Input: part model. Units: mm. Frame: model coordinates. A direction names the side the tool comes from. Coordinates: 2 decimals unless noted, no trailing zeros. Write each loop counter-clockwise with the first axis right and the second up, starting at its lowest first coordinate (ties: lowest second). Pieces come first, ordered by that corner, then holes. Notation, with made-up numbers: (13.25, 55) - (56.25, 55) arc R17 ccw to (56.25, 69) - close; hole circle Ø10 at (42, -19.75). An arc over 180 degrees is marked (long way). Put each result on its own line as item: value. Start each with the question number.
1. Access query for faces 4 (the flat face through (3, -63.586, -20)), 5 (the flat face through (2.96, -75.19, -37.71)), 6 (the flat face through (3, 14, -11.184)). Directions: +Z, -Z, +X, -X, +Y, -Y. A direction counts if a zero-diameter tool reaches every point of the face in a straight line with its end or side. Return the directions, or none.
2. Cut plane A-A, the plane x = 1.7. Count the separate pieces of the cut face and the enclosed holes in it, and give its area (3 significant figures).
3. Pin query (flat end, axial travel): pin 1 (1.8 mm diameter, centred on x = 1.5, z = -19.5, fed in from +Y); pin 2 (3 mm diameter, centred on x = 3.5, y = -78, fed in from -Z); pin 3 (3 mm diameter, centred on x = 3.5, y = 16.5, fed in from +Z). Return the tip coordinate at first contact, or that it passes through.
4. Cut plane D-D, the plane y = -15.5. Return loops of the section in (x, z).
5. Pull-direction query (Y, two-part tool) for faces 1 (the flat face through (3, -84.98, -9)), 2 (the flat face through (3, -75.586, 4)), 3 (the flat face through (3, 13, -29.184)); classes: released by +Y, released by -Y, zero draft, split by the parting line, or undercut.
6. Cut plane B-B, the plane z = -38. Return loops of the section in (x, y), and give its area (3 significant figures).
7. Line query: line 1 (Y direction, x = 3.5, z = 8.5); line 2 (Z direction, x = 2.75, y = 13); line 3 (Y direction, x = 1.3, z = 14). Output: solid intervals per line, ascending.
8. Cut plane C-C, the plane z = -12.5. Return loops of the section in (x, y), and give its area (3 significant figures).
from build123d import *

# Parameters (mm, degrees)
SKETCH1_W           = 12
SKETCH1_H           = 6
BOSS_EXTRUDE1_DEPTH = 6


with BuildPart() as part:
    # Sketch1 → Boss-Extrude1 (new body)
    with BuildSketch(Plane(origin=(0, 0, 0), x_dir=(0, 0, -1), z_dir=(1, 0, 0))):
        with BuildLine():
            Line((-19.809776263, 10.405108849), (-19.809776263, -84.98038082))
            Line((-19.809776263, -84.98038082), (39.507973257, -84.98038082))
            Line((39.507973257, -84.98038082), (35.862319142, -65.117665917))
            ThreePointArc((35.862319142, -65.117665917), (36.331936953, -30.24496444), (50.023720259, 1.830897499))
            Line((50.023720259, 1.830897499), (52.190223737, 5.008360642))
            Line((52.190223737, 5.008360642), (52.190223737, 10.405108849))
            Line((52.190223737, 10.405108849), (41.184188047, 10.405108849))
            Line((41.184188047, 10.405108849), (41.184188047, 16.405108849))
            Line((41.184188047, 16.405108849), (29.184188047, 16.405108849))
            Line((29.184188047, 16.405108849), (29.184188047, 10.405108849))
            Line((29.184188047, 10.405108849), (11.184188047, 10.405108849))
            Line((11.184188047, 10.405108849), (11.184188047, 18.63698455))
            Line((11.184188047, 18.63698455), (-0.815811953, 18.63698455))
            Line((-0.815811953, 18.63698455), (-0.815811953, 10.405108849))
            Line((-0.815811953, 10.405108849), (-19.809776263, 10.405108849))
        make_face()
        with Locations((-3.863115861, -78.586137139)):
            Rectangle(SKETCH1_W, SKETCH1_H, mode=Mode.SUBTRACT)
        with Locations((20.136884139, -78.586137139)):
            Rectangle(SKETCH1_W, SKETCH1_H, mode=Mode.SUBTRACT)
        with Locations((-3.863115861, -66.586137139)):
            Rectangle(SKETCH1_W, SKETCH1_H, mode=Mode.SUBTRACT)
        with Locations((20.136884139, -66.586137139)):
            Rectangle(SKETCH1_W, SKETCH1_H, mode=Mode.SUBTRACT)
    extrude(amount=BOSS_EXTRUDE1_DEPTH)


solid = part.part
Report:
1. face 4: +X, -X
1. face 5: -Z, +X, -X
1. face 6: +X, -X, +Y
2. separate pieces: 1
2. enclosed holes: 4
2. area: 5,530 mm^2
3. pin 1: stops at y = 10.41
3. pin 2: stops at z = -38.5
3. pin 3: stops at z = 0.82
4. outline: (0, -40.8) - (6, -40.8) - (6, 19.81) - (0, 19.81) - close
5. face 1: released by -Y
5. face 2: undercut
5. face 3: zero draft
6. outline: (0, -84.98) - (6, -84.98) - (6, -76.76) - (0, -76.76) - close; (0, -23.61) - (6, -23.61) - (6, 16.41) - (0, 16.41) - close
6. area: 289 mm^2
7. line 1: y = -84.98 to -81.59, -75.59 to -69.59, -63.59 to 10.41
7. line 2: z = -41.18 to -29.18, -11.18 to 0.82
7. line 3: y = -84.98 to 10.41
8. outline: (0, -84.98) - (6, -84.98) - (6, 10.41) - (0, 10.41) - close
8. area: 572 mm^2
